Check sheet for the modelled part. Datum: model origin and axes. Units: mm. Face numbers are marked on the shaded views. Round coordinates to 2 decimals unless told otherwise and drop trailing zeros. Write each loop counter-clockwise with the first axis right and the second up, starting at its lowest first coordinate (ties: lowest second). Pieces come first, ordered by that corner, then holes. Notation, with made-up numbers: (20, 16.25) -> (77, 16.25) arc R30 cw to (77, 53.25) -> close; hole circle Ø2 at (71, 43). An arc over 180 degrees is marked (long way). One line per item, written item: value.
from build123d import *

# Parameters (mm, degrees)
EXTRUDE_1_DEPTH     = 3
SKETCH_2_R          = 2.025
CUT_EXTRUDE_1_DEPTH = 3
FILLET_1_R          = 3


with BuildPart() as part:
    # 草图1 → 凸台-拉伸1 (new body)
    with BuildSketch(Plane.XY):
        Polygon((0, 0), (0, 50), (20, 50), (20, 20), (50, 20), (50, 0), align=None)
    extrude(amount=EXTRUDE_1_DEPTH)

    # 草图2 → 切除-拉伸1 (cut)
    with BuildSketch(Plane.XY.offset(3)):
        with Locations((10, 10)):
            Circle(SKETCH_2_R)
        with Locations((10, 44)):
            Circle(SKETCH_2_R)
        with Locations((44, 10)):
            Circle(SKETCH_2_R)
    extrude(amount=-CUT_EXTRUDE_1_DEPTH, mode=Mode.SUBTRACT)

    # 圆角1
    fillet_1_edges = [part.edges().sort_by_distance(p)[0] for p in [
        (0, 0, 1.5),
        (0, 50, 1.5),
        (20, 50, 1.5),
        (20, 20, 1.5),
        (50, 20, 1.5),
        (50, 0, 1.5),
    ]]
    fillet(fillet_1_edges, radius=FILLET_1_R)


solid = part.part
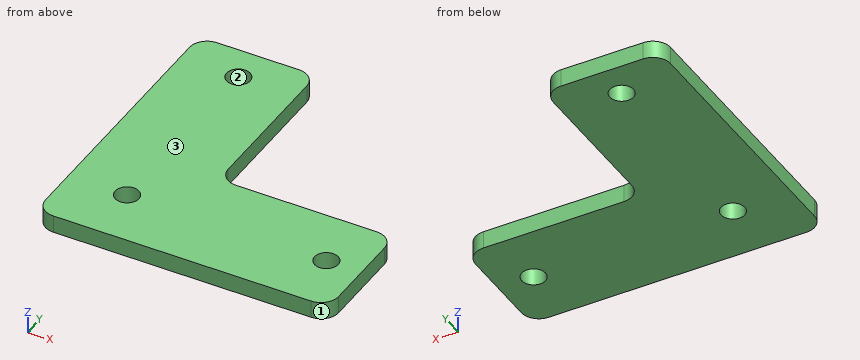
Item 1: Depth check by flat-ended pin: P1, Ø1, axis at x = 29.5, z = 2, coming from the +Y side; P2, Ø5.5, axis at x = 44, y = 10, coming from the +Z side; P3, Ø1.5, axis at y = 31, z = 1.5, coming from the +X side. Enter the tip coordinate at first touch or a pass-through.
Answer:
P1: stops at y = 20
P2: stops at z = 3
P3: stops at x = 20
Item 2: Sectioned sample at A-A on x = 10. Enter the section's corners in (y, z) (3 decimals), and give its area (3 significant figures).
Answer:
outline: (0, 0) -> (7.975, 0) -> (7.975, 3) -> (0, 3) -> close; (12.025, 0) -> (41.975, 0) -> (41.975, 3) -> (12.025, 3) -> close; (46.025, 0) -> (50, 0) -> (50, 3) -> (46.025, 3) -> close
area: 126 mm^2
Item 3: Mould release check, pull along Y, two halves, no side actions. Record for the marked faces 1, 2 and 3: pulls with the +Y half, pulls with the -Y half, needs draft (parallel to the pull), parting line crosses it, or undercut.
Answer:
face 1: pulls with the -Y half
face 2: undercut
face 3: needs draft
Item 4: Sectioned sample at B-B on z = 0.7. Enter the section's corners in (x, y) (3 decimals), and give its area (3 significant figures).
Answer:
outline: (0, 3) arc R3 ccw to (3, 0) -> (47, 0) arc R3 ccw to (50, 3) -> (50, 17) arc R3 ccw to (47, 20) -> (23, 20) arc R3 cw to (20, 23) -> (20, 47) arc R3 ccw to (17, 50) -> (3, 50) arc R3 ccw to (0, 47) -> close; hole circle Ø4.05 at (10, 10); hole circle Ø4.05 at (10, 44); hole circle Ø4.05 at (44, 10)
area: 1,550 mm^2
Item 5: Thickness scan on line 1 (Y direction, x = 10, z = 2.3) (3 decimals); line 2 (Y direction, x = 44, z = 0.95) (3 decimals); line 3 (Y direction, x = 11, z = 2.05). Record the ranges inside material, lowest first.
Answer:
line 1: y = 0 to 7.975, 12.025 to 41.975, 46.025 to 50
line 2: y = 0 to 7.975, 12.025 to 20
line 3: y = 0 to 8.24, 11.76 to 42.24, 45.76 to 50
Item 6: Sectioned sample at C-C on y = 44. Enter the section's corners in (x, z) (3 decimals), and give its area (4 significant figures).
Answer:
outline: (0, 0) -> (7.975, 0) -> (7.975, 3) -> (0, 3) -> close; (12.025, 0) -> (20, 0) -> (20, 3) -> (12.025, 3) -> close
area: 47.85 mm^2
